Verification items for the finished model (mm, model axes). A direction names the side the tool comes from. Round coordinates to 2 decimals unless told otherwise and drop trailing zeros. Loops run counter-clockwise (first coordinate to the right, second up) from the corner with the lowest first, then second, coordinate; pieces in that order, holes last. Notation, with made-up numbers: M -18.5,2.25 L 3.5,2.25 A16 ccw 3.5,32.25 Z; hole C 63,-16.75 d4. An arc over 180 degrees is marked long. Answer as CSV lines item,"result".
```python
from build123d import *

# Parameters (mm, degrees)
F0_W          = 5
F0_H          = 26
F1_ANGLE_BACK = 110
F1_ANGLE      = 220
F2_W          = 22
F2_H          = 26
F3_DEPTH      = 5
F3_DEPTH_BACK = 5
F4_R          = 2.49999
F5_W          = 15.8
F5_H          = 19.7
F6_DEPTH      = 10
F7_R          = 1.25
F8_DEPTH      = 42.901
F9_R          = 2
F10_R         = 5


# Not quite as in the source:
# - a fillet or chamfer is up to 0.001 mm smaller than in the source, because OpenCascade refuses the exact size


with BuildPart() as f1:
    # F0 (on Right) → F1 (revolve)
    with BuildSketch(Plane.YZ, mode=Mode.PRIVATE) as f1_sk:
        with Locations((2.5, 0)):
            Rectangle(F0_W, F0_H)
    revolve(f1_sk.sketch.rotate(Axis((0, 35, 2.8591789305), (0, 0, -1)), -F1_ANGLE_BACK), axis=Axis((0, 35, 2.8591789305), (0, 0, -1)), revolution_arc=F1_ANGLE)

    # F2 (on Front) → F3 (join, two sides)
    with BuildSketch(Plane.XZ) as f3_sk:
        Rectangle(F2_W, F2_H)
    extrude(amount=F3_DEPTH)
    extrude(f3_sk.sketch, amount=-F3_DEPTH_BACK)

    # F4 (radius 2.5 in the source; OpenCascade refuses exactly that, so slightly less here)
    f4_edges = [f1.edges().sort_by_distance(p)[0] for p in [
        (32.889242, 46.970705, 0),
        (28.190779, 45.260604, 0),
        (-28.190779, 45.260604, 0),
        (-32.889242, 46.970705, 0),
    ]]
    fillet(f4_edges, radius=F4_R)

    # F5 (on face) → F6 (join)
    with BuildSketch(Plane.XZ.offset(5)):
        Rectangle(F5_W, F5_H)
    extrude(amount=F6_DEPTH)

    # F7 (on face) → F8 (cut, through all)
    with BuildSketch(Plane.YZ.offset(7.9)):
        with Locations((-11, 5.85)):
            Circle(F7_R)
        with Locations((-11, -5.85)):
            Circle(F7_R)
    extrude(amount=-F8_DEPTH, mode=Mode.SUBTRACT)

    # F9
    f9_edges = [f1.edges().sort_by_distance(p)[0] for p in [
        (7.9, -10, 9.85),
        (7.9, -10, -9.85),
        (-7.9, -10, -9.85),
        (-7.9, -10, 9.85),
    ]]
    fillet(f9_edges, radius=F9_R)

    # F10
    f10_edges = [f1.edges().sort_by_distance(p)[0] for p in [
        (-11, -1.613248, 13),
        (-11, -1.613248, -13),
        (11, -1.613248, -13),
        (11, -1.613248, 13),
    ]]
    fillet(f10_edges, radius=F10_R)


solid = f1.part
```
1) Section check A-A (y = -11). Record the cut outline in (x, z), plus the area to 3 significant figures.
Here are the results:
outline,"M -7.9,-7.85 A2 ccw -5.9,-9.85 L 5.9,-9.85 A2 ccw 7.9,-7.85 L 7.9,-7.1 L -7.9,-7.1 Z; M -7.9,-4.6 L 7.9,-4.6 L 7.9,4.6 L -7.9,4.6 Z; M -7.9,7.1 L 7.9,7.1 L 7.9,7.85 A2 ccw 5.9,9.85 L -5.9,9.85 A2 ccw -7.9,7.85 Z"
area,"229 mm^2"
2) Set-up check for faces 1 (the cylindrical face through (9, -2, 12)), 2 (the flat face through (0, -10, 9.85)), 3 (the cylindrical face through (-10, -2, 11)), 4 (the flat face through (0, -10, -9.85)): record each of +Z, -Z, +X, -X, +Y, -Y from which the full face is reachable in a straight line by a thin tool's end or side.
Here are the results:
face 1,"+Z, +X, -Y"
face 2,"+Z, +X, -X, -Y"
face 3,"+Z, -X, -Y"
face 4,"-Z, +X, -X, -Y"
3) Material ranges on probe 1 along Z at (x, y) = (-2, -11); probe 2 along Y at (x, z) = (0, -1); probe 3 along X at (y, z) = (35, 3), recorded low to high.
Here are the results:
probe 1,"z = -9.85 to -7.1, -4.6 to 4.6, 7.1 to 9.85"
probe 2,"y = -15 to 5"
probe 3,"x = -35 to -30, 30 to 35"
4) Draft check along Z on faces 5 (the cylindrical face through (7.3, -10.07, -9.28)), 6 (the flat face through (5, 5, 13)), 7 (the cylindrical face through (0.111, -11.921, -5.005)). Enter one of: +Z half, -Z half, draft (parallel to the pull), parting line (faces both ways), or undercut.
Here are the results:
face 5,"-Z half"
face 6,"+Z half"
face 7,"undercut"
5) Section check B-B (y = 35). Record the cut outline in (x, z), plus the area to 3 significant figures.
Here are the results:
outline,"M -35,-13 L -30,-13 L -30,13 L -35,13 Z; M 30,-13 L 35,-13 L 35,13 L 30,13 Z"
area,"260 mm^2"
6) Go/stop test with flat-tipped pins: pin 1 (2 mm diameter, centred on y = -11, z = 5.85, fed in from -X); pin 2 (1.5 mm diameter, centred on y = 22.5, z = -8, fed in from +X); pin 3 (8 mm diameter, centred on y = -11, z = 0.5, fed in from +X); pin 4 (3 mm diameter, centred on y = -11, z = -5.85, fed in from -X). Record where each tip stops, or that it passes through.
Here are the results:
pin 1,"passes through"
pin 2,"stops at x = 32.97"
pin 3,"stops at x = 7.9"
pin 4,"stops at x = -7.9"
7) Section check D-D (x = 0). Record the cut outline in (y, z), plus the area to 3 significant figures.
Here are the results:
outline,"M -15,-9.85 L -5,-9.85 L -5,-13 L 5,-13 L 5,13 L -5,13 L -5,9.85 L -15,9.85 Z; hole C -11,-5.85 d2.5; hole C -11,5.85 d2.5"
area,"447 mm^2"
